from build123d import *

# Parameters (mm, degrees)
SKETCH1_W           = 127
SKETCH1_H           = 50.8
BOSS_EXTRUDE1_DEPTH = 12.7
CUT_EXTRUDE1_DEPTH  = 12.7


with BuildPart() as part:
    # Sketch1 → Boss-Extrude1 (new body)
    with BuildSketch(Plane(origin=(0, 0, 0), x_dir=(1, 0, 0), z_dir=(0, 1, 0))):
        with Locations((63.5, 25.4)):
            Rectangle(SKETCH1_W, SKETCH1_H)
    extrude(amount=BOSS_EXTRUDE1_DEPTH)

    # Sketch2 → Cut-Extrude1 (cut)
    with BuildSketch(Plane(origin=(0, 12.7, 0), x_dir=(1, 0, 0), z_dir=(0, 1, 0))):
        with BuildLine():
            ThreePointArc((9.125, 25), (13.774679849, 13.774679849), (25, 9.125))
            Line((25, 9.125), (25, 25))
            Line((25, 25), (9.125, 25))
        make_face()
        with BuildLine():
            Line((25, 25), (25, 9.125))
            ThreePointArc((25, 9.125), (36.225320151, 13.774679849), (40.875, 25))
            ThreePointArc((40.875, 25), (25, 40.875), (9.125, 25))
            Line((9.125, 25), (25, 25))
        make_face()
    extrude(amount=-CUT_EXTRUDE1_DEPTH, mode=Mode.SUBTRACT)


solid = part.part
Geometry check sheet. Reference: the model listing, model coordinates, mm. Round coordinates to 2 decimals unless told otherwise and drop trailing zeros. Write each loop counter-clockwise with the first axis right and the second up, starting at its lowest first coordinate (ties: lowest second). Pieces come first, ordered by that corner, then holes. Notation, with made-up numbers: (65.5, -36.75) -> (117.5, -36.75) arc R24 ccw to (117.5, -15.75) -> close; hole circle Ø9 at (55, 61.25). An arc over 180 degrees is marked (long way). One line per item, written item: value. Start each with the question number.
(1) Cross-section at B-B, the plane z = -14.5. Record the cut outline in (x, y).
(2) Scan lines: line 1 (X direction, y = 12, z = -17); line 2 (X direction, y = 10.5, z = -15); line 3 (Z direction, x = 30, y = 10.75). Record each from-to range of solid material in increasing order. Write a range as [from, to].
(3) Cross-section at A-A, the plane y = 10. Record the cut outline in (x, z) (3 decimals), and give its area (3 significant figures).
(4) Cross-section at C-C, the plane x = 29.5. Record the cut outline in (y, z).
Answer:
1. outline: (0, 0) -> (13.09, 0) -> (13.09, 12.7) -> (0, 12.7) -> close; (36.91, 0) -> (127, 0) -> (127, 12.7) -> (36.91, 12.7) -> close
2. line 1: [0, 11.29], [38.71, 127]
2. line 2: [0, 12.67], [37.33, 127]
2. line 3: [-50.8, -40.07], [-9.93, 0]
3. outline: (0, -50.8) -> (127, -50.8) -> (127, 0) -> (0, 0) -> close; hole circle Ø31.75 at (25, -25)
3. area: 5,660 mm²
4. outline: (0, -50.8) -> (12.7, -50.8) -> (12.7, -40.22) -> (0, -40.22) -> close; (0, -9.78) -> (12.7, -9.78) -> (12.7, 0) -> (0, 0) -> close
